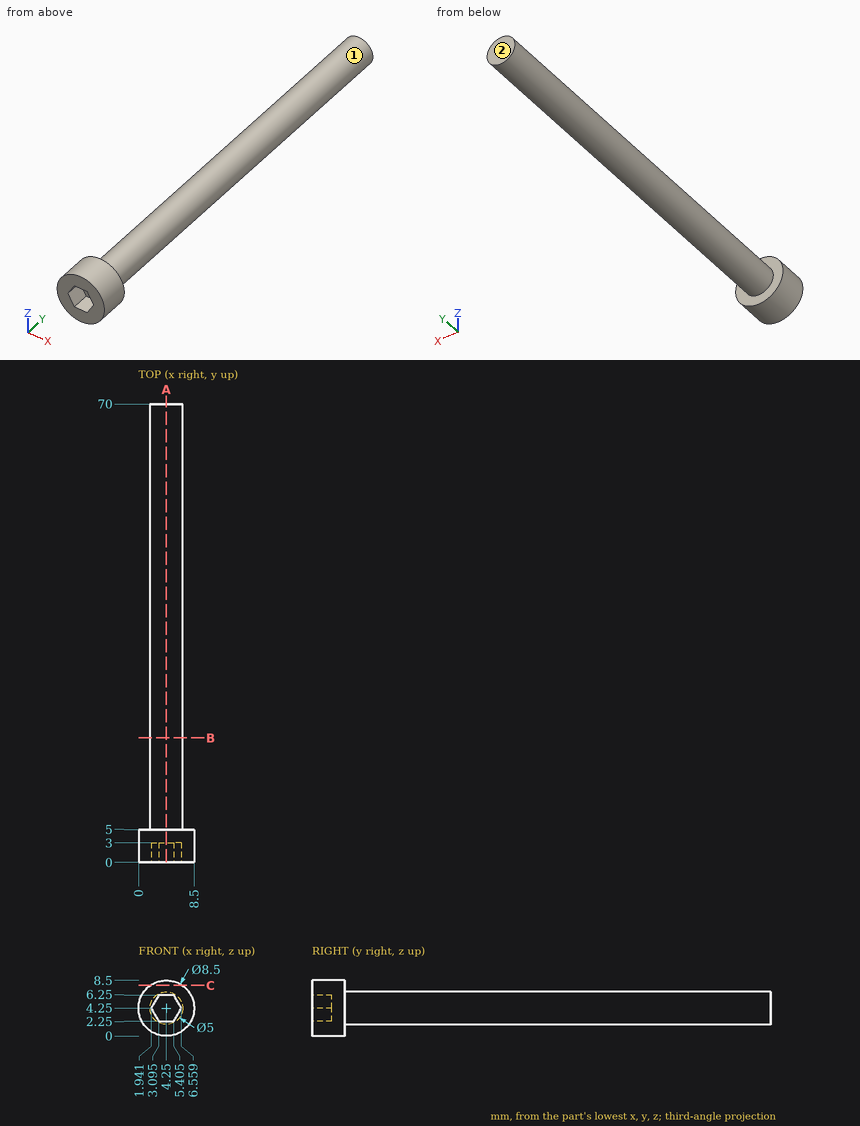
Study the drawing (mm; zero at the part's minimum x, y, z) and answer. A direction names the side the tool comes from. Give positions to 0.01 mm unless a question says otherwise; leave off trailing zeros. Loops run counter-clockwise (first coordinate to the right, second up) from the corner with the lowest first, then second, coordinate; pieces in that order, holes last. Notation, with made-up numbers: (-7.75, 73) - (33.25, 73) arc R13 cw to (33.25, 96) - close; hole circle Ø2 at (72.25, -17.5). An arc over 180 degrees is marked (long way). One line per question, with ' | ' between items.
(1) Each of these flat-tipped pins is pushed along its axis until it touches: pin 1 Ø1.5 at (x, y) = (5.5, 47.5) entering from -Z; pin 2 Ø3 at (x, y) = (4.5, 56) entering from +Z; pin 3 Ø3 at (y, z) = (10.5, 6) entering from -X. Where does it stop, or does it pass through?
Recorded:
pin 1: stops at z = 1.8 | pin 2: stops at z = 6.75 | pin 3: stops at x = 1.76
(2) A tool of negligible diameter and unlimited length cuts with its end or side. For the marked faces 1 and 2, from which of +Z, -Z, +X, -X, +Y, -Y can it reach the whole face along a straight path? Write none if from no direction.
Recorded:
face 1: +Y | face 2: +Z, -Z, +X, -X, +Y
(3) The part is cut by section B-B (y = 19). Write down the section's boundary in (x, z), then the cut area to 3 significant figures.
Recorded:
outline: circle Ø5 at (4.25, 4.25) | area: 19.6 mm²
(4) The part is cut by section A-A (x = 4.25). Write down the section's boundary in (y, z).
Recorded:
outline: (0, 0) - (5, 0) - (5, 1.75) - (70, 1.75) - (70, 6.75) - (5, 6.75) - (5, 8.5) - (0, 8.5) - (0, 6.25) - (3, 6.25) - (3, 2.25) - (0, 2.25) - close
(5) The part is cut by section C-C (z = 7.75). Write down the section's boundary in (x, y), then the cut area to 3 significant figures.
Recorded:
outline: (1.84, 0) - (6.66, 0) - (6.66, 5) - (1.84, 5) - close | area: 24.1 mm²
(6) Straight lines are drawn through the part: probe 1 along Y at (x, z) = (6, 1.5); probe 2 along X at (y, z) = (5.5, 4.25); probe 3 along Z at (x, y) = (4.5, 37). For each, find the intervals that lie inside material, in ascending order.
Recorded:
probe 1: y = 0 to 5 | probe 2: x = 1.75 to 6.75 | probe 3: z = 1.76 to 6.74
